Autodesk Inventor part; units mm, degrees
ref_plane "YZ Plane" through (0, 0, 0) normal (1, 0, 0) x (0, 1, 0)
ref_plane "XZ Plane" through (0, 0, 0) normal (0, 1, 0) x (-1, 0, 0)
ref_plane "XY Plane" through (0, 0, 0) normal (0, 0, 1) x (1, 0, 0)
sketch "スケッチ1" plane through (0, 0, 0) normal (0, 0, 1) x (1, 0, 0)
  circle A0 centre (0, 0) radius 7.5
  circle A1 centre (0, 0) radius 30
  circle A2 centre (0, 0) radius 37.5
  circle A3 centre (23.5425, -29.1891) radius 30
  circle A4 centre (23.5425, -29.1891) radius 4
  circle A5 centre (23.5425, -29.1891) radius 16
  circle A6 centre (23.5425, -29.1891) radius 56
  circle A7 centre (0, -80) radius 40
  circle A8 centre (0, -80) radius 50
  circle A9 centre (0, -80) radius 4
  dimension "d57" = 75
  dimension "d64" = 112
  dimension "d41" = 15
  dimension "d58" = 8
  dimension "d63" = 32
  dimension "d65" = 100
  dimension "d66" = 8
sketch "スケッチ2" plane through (0, 0, 0) normal (0, 0, 1) x (1, 0, 0)
  line L0 (0, 0) -> (24.502, 0) construction
  line L1 (0, 0) -> (12.5, 0) construction
  line L2 (0, 0) -> (10.253, 10.253)
  line L3 (0, 0) -> (14.5, 0) construction
  line L4 (10.253, 10.253) -> (-10.253, -10.253)
  circle A0 centre (10.253, 10.253) radius 2
  circle A1 centre (-10.253, -10.253) radius 2
  circle A2 centre (0, 0) radius 7.5
  line L5 (0, 0) -> (28.1908, 10.2606)
  line L6 (0, 0) -> (30, 0) construction
  line L7 (0, 0) -> (-28.1908, 10.2606)
  line L8 (0, 0) -> (30, 0) construction
  circle A3 centre (-28.1908, 10.2606) radius 2.5
  line L9 (0, 0) -> (0, 30)
  circle A4 centre (0, 30) radius 2.5
  circle A5 centre (28.1908, 10.2606) radius 2.5
  dimension "d9" = 14.5
  dimension "d10" = 45
  dimension "d11" = 29
  dimension "d12" = 4
  dimension "d13" = 4
  dimension "d14" = 15
  dimension "d15" = 30
  dimension "d16" = 20
  dimension "d17" = 30
  dimension "d18" = 160
  dimension "d19" = 5
  dimension "d20" = 30
  dimension "d21" = 5
  dimension "d22" = 5
sketch "スケッチ3" plane through (0, 0, 0) normal (0, 0, 1) x (1, 0, 0)
  line L0 (60, -99.3436) -> (-60, -99.3436)
  line L1 (-60, -99.3436) -> (-60, 99.3436)
  line L2 (-60, 99.3436) -> (60, 99.3436)
  line L3 (60, 99.3436) -> (60, -99.3436)
  line L4 (60, -99.3436) -> (-60, 99.3436) construction
  line L5 (-60, -99.3436) -> (60, 99.3436) construction
  point P0 (0, 0)
  dimension "d25" = 120
extrude "押し出し1" add sketch "スケッチ3" against normal blind 3
sketch "スケッチ4" plane through (0, 0, 0) normal (0, 0, 1) x (1, 0, 0)
  line L0 (0, 45.0711) -> (68.3595, 45.0711)
  line L1 (68.3595, 45.0711) -> (-74.3824, 45.0711)
  line L2 (-74.3824, 45.0711) -> (108.1656, 45.0711)
  line L3 (108.1656, 45.0711) -> (108.1656, 129.4154)
  line L4 (108.1656, 129.4154) -> (-74.3824, 129.4154)
  line L5 (-74.3824, 129.4154) -> (-74.3824, 45.0711)
  point P0 (0, 0)
extrude "押し出し4" cut sketch "スケッチ4" against normal blind 10
fillet "フィレット1" radius 4 4 edges at (-60, 45.0711, -1.5) (60, 45.0711, -1.5) (-60, -99.3436, -1.5) (60, -99.3436, -1.5)
extrude "押し出し9" cut sketch "スケッチ1" against normal blind 10 contours A4 A2 | A2 A4 | A9 A6 | A6 A9
sketch "スケッチ8" plane through (0, 0, 0) normal (0, 0, 1) x (1, 0, 0)
  line L0 (-265.6992, -158.784) -> (100.3409, -158.784)
  line L1 (100.3409, -158.784) -> (100.3409, -94)
  line L2 (100.3409, -94) -> (-265.6992, -94)
  line L3 (-265.6992, -94) -> (-265.6992, -158.784)
  line L4 (-265.6992, -158.784) -> (100.3409, -94) construction
  line L5 (100.3409, -158.784) -> (-265.6992, -94) construction
  point P0 (0, 0)
  point P1 (0, -94)
  point P2 (-82.6791, -126.392)
extrude "押し出し10" cut sketch "スケッチ8" against normal blind 10
extrude "押し出し11" cut sketch "スケッチ2" against normal blind 10 contours A5 | A3 | A4
sketch "スケッチ9" plane through (0, 0, 0) normal (0, 0, 1) x (1, 0, 0)
  circle A0 centre (-50, -84) radius 2
  circle A1 centre (50, -84) radius 2
  circle A2 centre (-50, -70) radius 2
  circle A3 centre (50, -70) radius 2
  point P0 (0, 0)
  dimension "d73" = 4
  dimension "d74" = 4
  dimension "d75" = 4
  dimension "d76" = 4
extrude "押し出し12" cut sketch "スケッチ9" against normal blind 10
sketch "スケッチ10" plane through (0, 0, -3) normal (0, 0, -1) x (-1, 0, 0)
  circle A0 centre (-23.5425, -29.1891) radius 4
  circle A1 centre (-23.5425, -29.1891) radius 11
  circle A2 centre (0, -80) radius 4
  circle A3 centre (0, -80) radius 11
  point P0 (0, 0)
  dimension "d79" = 22
  dimension "d80" = 22
extrude "押し出し13" cut sketch "スケッチ10" against normal blind 10
properties part number "板2" material "アルミニウム 6061"
Input: part model. Units: mm. Frame: model coordinates. Coordinates: 2 decimals unless noted, no trailing zeros. Write each loop counter-clockwise with the first axis right and the second up, starting at its lowest first coordinate (ties: lowest second). Pieces come first, ordered by that corner, then holes.
1) Section A-A on y = -80. Output: boundary loops of the cut face in (x, z).
2) Section C-C on x = 23. Output: boundary loops of the cut face in (y, z), and give its area (3 significant figures).
3) Section B-B on x = -50. Output: boundary loops of the cut face in (y, z).
4) Section D-D on z = -1.3. State how many separate pieces and enclosed holes the cut face has, and give its area (3 significant figures).
5) Mould query, pull axis X, two halves, no side actions, for faces 1 (the flat face through (-60, -27, -1)), 2 (the cylindrical face through (-50, -68, -1)), 3 (the flat face through (-1, -23, 0)), 4 (the cylindrical face through (1.432, -69.094, -1.521)). Classes: pulls with the +X half, pulls with the -X half, needs draft (parallel to the pull), parting line crosses it, or undercut.
6) Material intervals for line 1 along Y through (x, z) = (-50, -1.65); line 2 along Y through (x, z) = (27, -2.9); line 3 along Y through (x, z) = (-4, -1), sorted ascending.
Check result:
1. outline: (-60, -3) - (-11, -3) - (-11, 0) - (-60, 0) - close; (11, -3) - (60, -3) - (60, 0) - (11, 0) - close
2. outline: (-94, -3) - (-40.18, -3) - (-40.18, 0) - (-94, 0) - close; (-18.2, -3) - (45.07, -3) - (45.07, 0) - (-18.2, 0) - close
2. area: 351 mm2
3. outline: (-94, -3) - (-86, -3) - (-86, 0) - (-94, 0) - close; (-82, -3) - (-72, -3) - (-72, 0) - (-82, 0) - close; (-68, -3) - (45.07, -3) - (45.07, 0) - (-68, 0) - close
4. separate pieces: 1
4. enclosed holes: 9
4. area: 15,800 mm2
5. face 1: pulls with the -X half
5. face 2: undercut
5. face 3: needs draft
5. face 4: undercut
6. line 1: y = -94 to -86, -82 to -72, -68 to 45.07
6. line 2: y = -94 to -39.63, -18.75 to 8.06, 12.46 to 45.07
6. line 3: y = -94 to -90.25, -69.75 to 45.07
